from build123d import *

# Parameters (mm, degrees)
SKETCH1_W           = 213
SKETCH1_H           = 119.6
SKETCH1_R           = 1.5
SKETCH1_R_2         = 1.499999994
SKETCH1_R_3         = 2
SKETCH1_R_4         = 2.000000002
SKETCH1_R_5         = 5
BOSS_EXTRUDE1_DEPTH = 4
SKETCH5_R           = 1.5
SKETCH5_R_2         = 2
SKETCH5_RX          = 5.303428227
SKETCH5_RY          = 2
CUT_EXTRUDE1_DEPTH  = 4
SKETCH6_R           = 3
CUT_EXTRUDE2_DEPTH  = 4
SKETCH7_W           = 109
SKETCH7_H           = 3.522810192
SKETCH7_W_2         = 6
SKETCH7_H_2         = 119.6
SKETCH7_W_3         = 82.957650312
BOSS_EXTRUDE2_DEPTH = 4
FILLET7_R           = 1.5
FILLET8_R           = 8
FILLET9_R           = 8
FILLET10_R          = 8
FILLET11_R          = 8


with BuildPart() as part:
    # Sketch1 → Boss-Extrude1 (new body)
    with BuildSketch(Plane(origin=(0, 0, 0), x_dir=(1, 0, 0), z_dir=(0, 1, 0))):
        with Locations((106.5, 59.8)):
            Rectangle(SKETCH1_W, SKETCH1_H)
        with Locations((12, 93.6)):
            Circle(SKETCH1_R, mode=Mode.SUBTRACT)
        with Locations((12.113582234, 33.600107508)):
            Circle(SKETCH1_R, mode=Mode.SUBTRACT)
        with Locations((92, 93.6)):
            Circle(SKETCH1_R_2, mode=Mode.SUBTRACT)
        with Locations((92.113582234, 33.600107508)):
            Circle(SKETCH1_R, mode=Mode.SUBTRACT)
        with Locations((87.5, 103.6)):
            Circle(SKETCH1_R_2, mode=Mode.SUBTRACT)
        with Locations((102, 77.8)):
            Circle(SKETCH1_R_2, mode=Mode.SUBTRACT)
        with Locations((82.5, 103.6)):
            Circle(SKETCH1_R_2, mode=Mode.SUBTRACT)
        with Locations((77.5, 103.6)):
            Circle(SKETCH1_R_2, mode=Mode.SUBTRACT)
        with Locations((72.5, 103.6)):
            Circle(SKETCH1_R_2, mode=Mode.SUBTRACT)
        with Locations((67.5, 103.6)):
            Circle(SKETCH1_R_2, mode=Mode.SUBTRACT)
        with Locations((62.5, 103.6)):
            Circle(SKETCH1_R_2, mode=Mode.SUBTRACT)
        with Locations((57.5, 103.6)):
            Circle(SKETCH1_R_2, mode=Mode.SUBTRACT)
        with Locations((52.5, 103.6)):
            Circle(SKETCH1_R_2, mode=Mode.SUBTRACT)
        with Locations((102, 72.8)):
            Circle(SKETCH1_R_2, mode=Mode.SUBTRACT)
        with Locations((102, 67.8)):
            Circle(SKETCH1_R_2, mode=Mode.SUBTRACT)
        with Locations((102, 62.8)):
            Circle(SKETCH1_R_2, mode=Mode.SUBTRACT)
        with Locations((102, 57.8)):
            Circle(SKETCH1_R_2, mode=Mode.SUBTRACT)
        with Locations((102, 52.8)):
            Circle(SKETCH1_R_2, mode=Mode.SUBTRACT)
        with Locations((102, 47.8)):
            Circle(SKETCH1_R_2, mode=Mode.SUBTRACT)
        with Locations((102, 42.8)):
            Circle(SKETCH1_R_2, mode=Mode.SUBTRACT)
        with Locations((122, 93.6)):
            Circle(SKETCH1_R, mode=Mode.SUBTRACT)
        with Locations((155, 93.6)):
            Circle(SKETCH1_R, mode=Mode.SUBTRACT)
        with Locations((122, 34.6)):
            Circle(SKETCH1_R, mode=Mode.SUBTRACT)
        with Locations((155, 34.6)):
            Circle(SKETCH1_R, mode=Mode.SUBTRACT)
        with Locations((15.113582234, 23.600107508)):
            Circle(SKETCH1_R, mode=Mode.SUBTRACT)
        with Locations((20.137829951, 23.600107508)):
            Circle(SKETCH1_R, mode=Mode.SUBTRACT)
        with Locations((25.162077668, 23.600107508)):
            Circle(SKETCH1_R, mode=Mode.SUBTRACT)
        with Locations((30.186325385, 23.600107508)):
            Circle(SKETCH1_R, mode=Mode.SUBTRACT)
        with Locations((36.186325385, 23.600107508)):
            Circle(SKETCH1_R, mode=Mode.SUBTRACT)
        with Locations((41.186325385, 23.600107508)):
            Circle(SKETCH1_R, mode=Mode.SUBTRACT)
        with Locations((137.5, 101.6)):
            Circle(SKETCH1_R_3, mode=Mode.SUBTRACT)
        with Locations((142.5, 101.6)):
            Circle(SKETCH1_R_4, mode=Mode.SUBTRACT)
        with Locations((137.5, 26.6)):
            Circle(SKETCH1_R_3, mode=Mode.SUBTRACT)
        with Locations((142.5, 26.6)):
            Circle(SKETCH1_R_3, mode=Mode.SUBTRACT)
        with Locations((9, 110.6)):
            Circle(SKETCH1_R_5, mode=Mode.SUBTRACT)
        with Locations((9, 9)):
            Circle(SKETCH1_R_5, mode=Mode.SUBTRACT)
        with Locations((204, 110.6)):
            Circle(SKETCH1_R_5, mode=Mode.SUBTRACT)
        with Locations((204, 9)):
            Circle(SKETCH1_R_5, mode=Mode.SUBTRACT)
    extrude(amount=BOSS_EXTRUDE1_DEPTH)

    # Sketch5 → Cut-Extrude1 (cut)
    with BuildSketch(Plane(origin=(0, 4, 0), x_dir=(1, 0, 0), z_dir=(0, 1, 0))):
        with Locations((199.004449887, 99.6)):
            Circle(SKETCH5_R)
        with Locations((199.006879067, 73.600000113)):
            Circle(SKETCH5_R)
        with Locations((163.004450044, 99.596636519)):
            Circle(SKETCH5_R)
        with Locations((163.006879224, 73.596636633)):
            Circle(SKETCH5_R)
        with Locations((172.5, 107.84619775)):
            Circle(SKETCH5_R_2)
        with Locations((179.5, 107.84619775)):
            Circle(SKETCH5_R_2)
        with Locations((172.506879224, 65.346636633)):
            Circle(SKETCH5_R_2)
        with Locations((179.506879224, 65.346636633)):
            Circle(SKETCH5_R_2)
        with Locations((199.011329111, 45.999999887)):
            Circle(SKETCH5_R)
        with Locations((199.013758291, 20)):
            Circle(SKETCH5_R)
        with Locations((163.011329268, 45.996636406)):
            Circle(SKETCH5_R)
        with Locations((163.013758448, 19.996636519)):
            Circle(SKETCH5_R)
        with Locations((172.506879224, 54.246197637)):
            Circle(SKETCH5_R_2)
        with Locations((179.506879224, 54.246197637)):
            Circle(SKETCH5_R_2)
        with Locations((172.513758448, 11.746636519)):
            Circle(SKETCH5_R_2)
        with Locations((179.513758448, 11.746636519)):
            Circle(SKETCH5_R_2)
        with Locations(Location((207.004450044, 86.596636519), (0, 0, -90))):
            Ellipse(SKETCH5_RX, SKETCH5_RY)
        with Locations(Location((207.011329268, 32.996636406), (0, 0, -90))):
            Ellipse(SKETCH5_RX, SKETCH5_RY)
    extrude(amount=-CUT_EXTRUDE1_DEPTH, mode=Mode.SUBTRACT)

    # Sketch6 → Cut-Extrude2 (cut)
    with BuildSketch(Plane(origin=(0, 4, 0), x_dir=(1, 0, 0), z_dir=(0, 1, 0))):
        with Locations((42.5, 103.6)):
            Circle(SKETCH6_R)
    extrude(amount=-CUT_EXTRUDE2_DEPTH, mode=Mode.SUBTRACT)

    # Sketch7 → Boss-Extrude2 (add)
    with BuildSketch(Plane.XZ):
        with Locations((54.5, -84.838594904)):
            Rectangle(SKETCH7_W, SKETCH7_H)
        with Locations((112, -59.8)):
            Rectangle(SKETCH7_W_2, SKETCH7_H_2)
        with Locations((156.478825156, -84.838594904)):
            Rectangle(SKETCH7_W_3, SKETCH7_H)
    extrude(amount=BOSS_EXTRUDE2_DEPTH)

    # Fillet7
    fillet7_edges = [part.edges().sort_by_distance(p)[0] for p in [
        (0, -4, -84.838594904),
        (54.5, -4, -86.6),
        (115, -4, -103.1),
        (197.957650312, -4, -84.838594904),
        (156.478825156, -4, -83.077189808),
        (115, -4, -41.538594904),
        (112, -4, 0),
        (109, -4, -103.1),
        (112, -4, -119.6),
        (156.478825156, -4, -86.6),
        (109, -4, -41.538594904),
        (54.5, -4, -83.077189808),
    ]]
    fillet(fillet7_edges, radius=FILLET7_R)

    # Fillet8
    fillet8_edges = [part.edges().sort_by_distance(p)[0] for p in [
        (0, 2, -119.6),
    ]]
    fillet(fillet8_edges, radius=FILLET8_R)

    # Fillet9
    fillet9_edges = [part.edges().sort_by_distance(p)[0] for p in [
        (213, 2, -119.6),
    ]]
    fillet(fillet9_edges, radius=FILLET9_R)

    # Fillet10
    fillet10_edges = [part.edges().sort_by_distance(p)[0] for p in [
        (213, 2, 0),
    ]]
    fillet(fillet10_edges, radius=FILLET10_R)

    # Fillet11
    fillet11_edges = [part.edges().sort_by_distance(p)[0] for p in [
        (0, 2, 0),
    ]]
    fillet(fillet11_edges, radius=FILLET11_R)


solid = part.part
Geometry: final body of the model. Coordinates: model frame, mm. A direction names the side the tool comes from. Give positions to 0.01 mm unless a question says otherwise; leave off trailing zeros. Loops run counter-clockwise (first coordinate to the right, second up) from the corner with the lowest first, then second, coordinate; pieces in that order, holes last. Notation, with made-up numbers: M 74.5,58.5 L 98.5,58.5 A16 cw 98.5,79.5 Z; hole C 59,56.25 d3. An arc over 180 degrees is marked long. Put each result on its own line as item: value. Start each with the question number.
1) Ray query, line 1 along X through (y, z) = (0.5, -73); line 2 along Z through (x, y) = (77.5, 1.25); line 3 along Z through (x, y) = (122, 2.75). Return the intervals inside material, ascending.
2) Cut plane A-A (x = 142.5). Output: boundary loops of the cut face in (y, z).
3) Pull-direction query (Z, two-part tool) for faces 1 (the cylindrical face through (2.406, 2.028, -2.281)), 2 (the flat face through (105, 4, -61)), 3 (the cylindrical face through (177.5, 2, -107.9)); classes: pulls with the +Z half, pulls with the -Z half, needs draft (parallel to the pull), parting line crosses it, or undercut.
4) Contact query for flat-ended pins moving along their axis: pin 1 (2.5 mm diameter, centred on x = 179.5, z = -107.85, fed in from +Y); pin 2 (0.8 mm diameter, centred on x = 58.5, y = -1, fed in from +Z); pin 3 (1.5 mm diameter, centred on y = -3, z = -99.5, fed in from -X); pin 4 (1.5 mm diameter, centred on x = 158, z = -107, fed in from -Y). Output: stop coordinate, or through.
5) Access query for faces 4 (the flat face through (54, 0, -42)), 5 (the cylindrical face through (170.92, 2.03, -64.13)). Directions: +Z, -Z, +X, -X, +Y, -Y. A direction counts if a zero-diameter tool reaches every point of the face in a straight line with its end or side. Return the directions, or none.
6) Cut plane B-B (y = 2). Give the number of separate pieces and of enclosed holes in the cut face, then the cut area to 3 significant figures.
Verdict:
1. line 1: 0 to 100.51, 103.49 to 161.63, 164.38 to 197.63, 200.38 to 213
1. line 2: -119.6 to -105.1, -102.1 to 0
1. line 3: -119.6 to -95.1, -92.1 to -36.1, -33.1 to 0
2. outline: M -4,-85.1 A1.5 ccw -2.5,-86.6 L 0,-86.6 L 0,-99.6 L 4,-99.6 L 4,-28.6 L 0,-28.6 L 0,-83.08 L -2.5,-83.08 A1.5 ccw -4,-84.58 Z; M 0,-119.6 L 4,-119.6 L 4,-103.6 L 0,-103.6 Z; M 0,-24.6 L 4,-24.6 L 4,0 L 0,0 Z
3. face 1: pulls with the +Z half
3. face 2: needs draft
3. face 3: undercut
4. pin 1: through
4. pin 2: z = -83.08
4. pin 3: x = 109
4. pin 4: y = 0
5. face 4: +Z, -X, -Y
5. face 5: +Y, -Y
6. separate pieces: 1
6. enclosed holes: 57
6. area: 24,600 mm2
